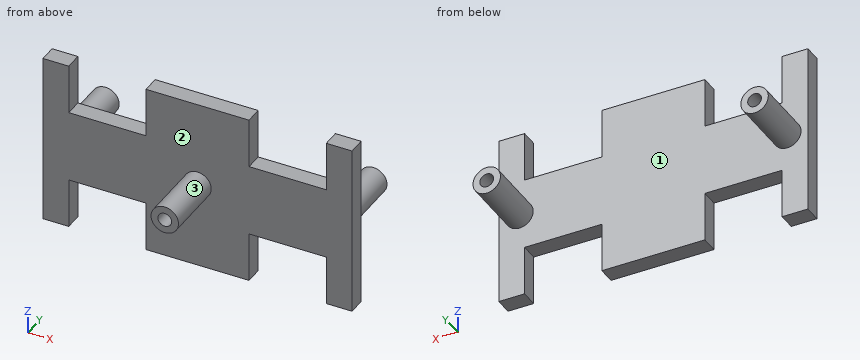
```python
from build123d import *

# Parameters (mm, degrees)
SKETCH3_W            = 90
SKETCH3_H            = 50
BOSS_EXTRUDE1_DEPTH  = 5
CUT_EXTRUDE1_DEPTH   = 5
MIRROR2_COPY_1_DEPTH = 5
SKETCH5_R            = 4
BOSS_EXTRUDE2_DEPTH  = 18
SKETCH6_R            = 2
CUT_EXTRUDE2_DEPTH   = 18
SKETCH8_R            = 4
BOSS_EXTRUDE3_DEPTH  = 18
SKETCH9_R            = 2
CUT_EXTRUDE3_DEPTH   = 18


with BuildPart() as part:
    # Sketch3 → Boss-Extrude1 (new body)
    with BuildSketch(Plane(origin=(0, 0, 0), x_dir=(1, 0, 0), z_dir=(0, 1, 0))):
        with Locations((-74.593596059, 13.903940887)):
            Rectangle(SKETCH3_W, SKETCH3_H)
    extrude(amount=BOSS_EXTRUDE1_DEPTH)

    # Sketch4 → Cut-Extrude1 (cut)
    with BuildSketch(Plane(origin=(0, 5, 0), x_dir=(1, 0, 0), z_dir=(0, 1, 0))):
        Polygon((-90.093596059, 24.403940887), (-89.593596059, 24.403940887), (-89.593596059, 38.903940887), (-112.093596059, 38.903940887), (-112.093596059, 24.403940887), align=None)
    cut_extrude1 = extrude(amount=-CUT_EXTRUDE1_DEPTH, mode=Mode.SUBTRACT)

    # Mirror1: Cut-Extrude1 across plane
    add(cut_extrude1.mirror(Plane.XY.offset(-13.903940887)), mode=Mode.SUBTRACT)

    # Mirror2: Cut-Extrude1 across plane
    add(cut_extrude1.mirror(Plane.ZY.offset(74.593596059)), mode=Mode.SUBTRACT)

    # Mirror2 copy 1 sketch → Mirror2 copy 1 (cut)
    with BuildSketch(Plane(origin=(-149.187192118, 5, -27.807881773), x_dir=(-1, 0, 0), z_dir=(0, 1, 0))):
        Polygon((-90.093596059, 24.403940887), (-89.593596059, 24.403940887), (-89.593596059, 38.903940887), (-112.093596059, 38.903940887), (-112.093596059, 24.403940887), align=None)
    extrude(amount=-MIRROR2_COPY_1_DEPTH, mode=Mode.SUBTRACT)

    # Sketch5 → Boss-Extrude2 (add)
    with BuildSketch(Plane(origin=(0, 5, 0), x_dir=(1, 0, 0), z_dir=(0, 1, 0))):
        with Locations(Location((-35.593596059, 13.903940887, 0), (0, 0, 270))):
            Circle(SKETCH5_R)
    boss_extrude2 = extrude(amount=BOSS_EXTRUDE2_DEPTH)

    # Sketch6 → Cut-Extrude2 (cut)
    with BuildSketch(Plane(origin=(0, 23, 0), x_dir=(1, 0, 0), z_dir=(0, 1, 0))):
        with Locations(Location((-35.593596059, 13.903940887, 0), (0, 0, 270))):
            Circle(SKETCH6_R)
    cut_extrude2 = extrude(amount=-CUT_EXTRUDE2_DEPTH, mode=Mode.SUBTRACT)

    # Mirror4: Boss-Extrude2, Cut-Extrude2 across plane
    add(boss_extrude2.mirror(Plane.ZY.offset(74.593596059)))
    add(cut_extrude2.mirror(Plane.ZY.offset(74.593596059)), mode=Mode.SUBTRACT)

    # Sketch8 → Boss-Extrude3 (add)
    with BuildSketch(Plane(origin=(0, 0, 0), x_dir=(-1, 0, 0), z_dir=(0, -1, 0))):
        with Locations(Location((74.593596059, 13.903940887, 0), (0, 0, 270))):
            Circle(SKETCH8_R)
    extrude(amount=BOSS_EXTRUDE3_DEPTH)

    # Sketch9 → Cut-Extrude3 (cut)
    with BuildSketch(Plane(origin=(0, -18, 0), x_dir=(-1, 0, 0), z_dir=(0, -1, 0))):
        with Locations(Location((74.593596059, 13.903940887, 0), (0, 0, 90))):
            Circle(SKETCH9_R)
    extrude(amount=-CUT_EXTRUDE3_DEPTH, mode=Mode.SUBTRACT)


solid = part.part
```
Part model, mm, in its own coordinate system. Face numbers are marked on the shaded views. Round coordinates to 2 decimals unless told otherwise and drop trailing zeros. Order: outer loops, then holes, each group sorted by start corner. A loop starts at its lowest first (then second) coordinate and runs counter-clockwise, first axis right, second up. Notation, with made-up numbers: M 54.25,52 L 110.25,52 A16 ccw 110.25,58 Z; hole C -30.75,8 d10. An arc over 180 degrees is marked long. Put each result on its own line as item: value. Start each with the question number.
1. Slice it at C-C on x = -102.5. List the corners of the cut face in (y, z), then the cut area to 3 significant figures.
2. Two-plate mould, pull along X, no slides. Class the marked faces 1, 2 and 3: +X half, -X half, draft (parallel to the pull), parting line (faces both ways), or undercut.
3. Slice it at D-D on y = 4. List the corners of the cut face in (x, z), then the cut area to 4 significant figures.
4. Slice it at A-A on z = 4. List the corners of the cut face in (x, y).
5. Slice it at B-B on y = 17.5. List the corners of the cut face in (x, z).
6. Drill centre lines: probe 1 along X at (y, z) = (4.5, -34); probe 2 along Y at (x, z) = (-113, -14); probe 3 along X at (y, z) = (10.5, -13). Where is each one in solid material? Low to high. Write a range as [from, to].
7. Drop flat-ended pins along their axis: pin 1 (4 mm diameter, centred on x = -61, z = -17.5, fed in from -Y); pin 2 (5.5 mm diameter, centred on x = -50.5, y = 2.5, fed in from -Z); pin 3 (4 mm diameter, centred on x = -40.5, z = -10, fed in from +Y); pin 4 (6.5 mm diameter, centred on x = -74.59, z = -13.9, fed in from -Y). Give the stop position or say it passes through.
Findings:
1. outline: M 0,-24.4 L 5,-24.4 L 5,-3.4 L 0,-3.4 Z
1. area: 105 mm2
2. face 1: undercut
2. face 2: draft
2. face 3: parting line
3. outline: M -119.59,-38.9 L -112.09,-38.9 L -112.09,-24.4 L -89.59,-24.4 L -89.59,-38.9 L -59.59,-38.9 L -59.59,-24.4 L -37.09,-24.4 L -37.09,-38.9 L -29.59,-38.9 L -29.59,11.1 L -37.09,11.1 L -37.09,-3.4 L -59.59,-3.4 L -59.59,11.1 L -89.59,11.1 L -89.59,-3.4 L -112.09,-3.4 L -112.09,11.1 L -119.59,11.1 Z
3. area: 3,195 mm2
4. outline: M -119.59,0 L -112.09,0 L -112.09,5 L -119.59,5 Z; M -89.59,0 L -59.59,0 L -59.59,5 L -89.59,5 Z; M -37.09,0 L -29.59,0 L -29.59,5 L -37.09,5 Z
5. outline: C -113.59,-13.9 d8; C -35.59,-13.9 d8; hole C -113.59,-13.9 d4; hole C -35.59,-13.9 d4
6. probe 1: [-119.59, -112.09], [-89.59, -59.59], [-37.09, -29.59]
6. probe 2: [0, 5]
6. probe 3: [-117.49, -115.38], [-111.81, -109.7], [-39.49, -37.38], [-33.81, -31.7]
7. pin 1: y = 0
7. pin 2: z = -24.4
7. pin 3: y = 5
7. pin 4: y = -18
